from build123d import *

# Parameters (mm, degrees)
SKETCH_1_W      = 10.2
SKETCH_1_H      = 13
EXTRUDE_1_DEPTH = 2.5
SKETCH_2_R      = 7.5
EXTRUDE_2_DEPTH = 2.9


with BuildPart() as part:
    # 草图1 → 凸台-拉伸1 (new body)
    with BuildSketch(Plane.XY):
        with Locations((-5.1, 6.5)):
            Rectangle(SKETCH_1_W, SKETCH_1_H)
    extrude(amount=EXTRUDE_1_DEPTH)

    # 草图2 → 凸台-拉伸2 (add)
    with BuildSketch(Plane.XY.offset(2.5)):
        with Locations(Location((-10.2, 6.5, 0), (0, 0, 299.926434867))):
            Circle(SKETCH_2_R)
    extrude(amount=EXTRUDE_2_DEPTH)


solid = part.part
Check sheet for the modelled part. Datum: model origin and axes. Units: mm. A direction names the side the tool comes from. Round coordinates to 2 decimals unless told otherwise and drop trailing zeros. Loops run counter-clockwise (first coordinate to the right, second up) from the corner with the lowest first, then second, coordinate; pieces in that order, holes last. Notation, with made-up numbers: M 27,6.25 L 76,6.25 A29 cw 76,34.25 Z; hole C 81,58.5 d1. An arc over 180 degrees is marked long. One line per question, with ' | ' between items. Start each with the question number.
Item 1: Set-up check for faces 1 (the face through (-5, 13, 1)), 2 (the face through (-5, 0, 1)), 3 (the face through (-9.233, -0.937, 3.93)): record each of +Z, -Z, +X, -X, +Y, -Y from which the full face is reachable in a straight line by a thin tool's end or side.
Item 2: Section check C-C (y = 11). Record the boundary of the cut face in (x, z), and give its area (3 significant figures).
Item 3: Gauge pin test, flat ends, axial feed: pin 1 Ø2 at (x, z) = (-6, 1) entering from -Y; pin 2 Ø3 at (y, z) = (11.5, 4) entering from -X; pin 3 Ø3.5 at (x, y) = (-13.5, 7.5) entering from -Z. Record the tip position at first contact, or that the pin passes through.
Item 4: Scan lines: probe 1 along Z at (x, y) = (-16, 4); probe 2 along Z at (x, y) = (-4.5, 0.75); probe 3 along X at (y, z) = (1.25, 1.35). Record each from-to range of solid material in increasing order.
Item 5: Section check D-D (x = -10.5). Record the boundary of the cut face in (y, z).
Item 6: Section check B-B (z = 3). Record the boundary of the cut face in (x, y).
Item 7: Section check A-A (y = 12.5). Record the boundary of the cut face in (x, z).
Worked out:
1) face 1: -Z, +X, -X, +Y | face 2: -Z, +X, -X, -Y | face 3: +Z
2) outline: M -16.2,2.5 L -10.2,2.5 L -10.2,0 L 0,0 L 0,2.5 L -4.2,2.5 L -4.2,5.4 L -16.2,5.4 Z | area: 60.3 mm^2
3) pin 1: y = 0 | pin 2: x = -16.83 | pin 3: z = 2.5
4) probe 1: 2.5 to 5.4 | probe 2: 0 to 2.5 | probe 3: -10.2 to 0
5) outline: M -0.99,2.5 L 13.99,2.5 L 13.99,5.4 L -0.99,5.4 Z
6) outline: C -10.2,6.5 d15
7) outline: M -14.7,2.5 L -10.2,2.5 L -10.2,0 L 0,0 L 0,2.5 L -5.7,2.5 L -5.7,5.4 L -14.7,5.4 Z
